from build123d import *

# Parameters (mm, degrees)
SKETCH1_W           = 260
SKETCH1_H           = 116
BOSS_EXTRUDE1_DEPTH = 75
SKETCH2_R           = 26.5
SKETCH2_W           = 191
SKETCH2_H           = 29
SKETCH2_H_2         = 77
SKETCH2_W_2         = 60
SKETCH2_H_3         = 25.123653406
SKETCH2_H_4         = 25.23272894
CUT_EXTRUDE1_DEPTH  = 69
FILLET1_R           = 5
FILLET2_R           = 5
SKETCH4_W           = 11.43
SKETCH4_H           = 4
CUT_EXTRUDE3_DEPTH  = 26.67
FILLET3_R           = 3
SKETCH5_W           = 55
SKETCH5_H           = 3
CUT_EXTRUDE4_DEPTH  = 1.5
SKETCH6_W           = 55
SKETCH6_H           = 3
CUT_EXTRUDE5_DEPTH  = 1.5
FILLET4_R           = 3
SKETCH7_W           = 162.299
SKETCH7_H           = 39.878
CUT_EXTRUDE6_DEPTH  = 10
SKETCH9_W           = 20
SKETCH9_H           = 3
CUT_EXTRUDE7_DEPTH  = 14.7
SKETCH10_W          = 3
SKETCH10_H          = 15.6
CUT_EXTRUDE8_DEPTH  = 22.8
SKETCH11_W          = 3
SKETCH11_H          = 22.8
BOSS_EXTRUDE2_DEPTH = 6.5
SKETCH12_W          = 15.39
SKETCH12_H          = 22.8
BOSS_EXTRUDE3_DEPTH = 3
SKETCH13_R          = 12.5
CUT_EXTRUDE9_DEPTH  = 3


with BuildPart() as part:
    # Sketch1 → Boss-Extrude1 (new body)
    with BuildSketch(Plane(origin=(0, 0, 0), x_dir=(1, 0, 0), z_dir=(0, 1, 0))):
        with Locations((130, 58)):
            Rectangle(SKETCH1_W, SKETCH1_H)
    extrude(amount=BOSS_EXTRUDE1_DEPTH)

    # Sketch2 → Cut-Extrude1 (cut)
    with BuildSketch(Plane(origin=(0, 75, 0), x_dir=(1, 0, 0), z_dir=(0, 1, 0))):
        with Locations((35, 58)):
            Circle(SKETCH2_R)
        with Locations((161.5, 98.5)):
            Rectangle(SKETCH2_W, SKETCH2_H)
        with Locations((161.5, 41.5)):
            Rectangle(SKETCH2_W, SKETCH2_H_2)
        with Locations((33, 100.438173297)):
            Rectangle(SKETCH2_W_2, SKETCH2_H_3)
        with Locations((33, 15.61636447)):
            Rectangle(SKETCH2_W_2, SKETCH2_H_4)
    extrude(amount=-CUT_EXTRUDE1_DEPTH, mode=Mode.SUBTRACT)

    # Fillet1
    fillet1_edges = [part.edges().sort_by_distance(p)[0] for p in [
        (0, 37.5, -116),
        (260, 37.5, -116),
        (260, 37.5, 0),
        (0, 37.5, 0),
    ]]
    fillet(fillet1_edges, radius=FILLET1_R)

    # Fillet2
    fillet2_edges = [part.edges().sort_by_distance(p)[0] for p in [
        (130, 0, -116),
        (0, 0, -58),
        (260, 0, -58),
        (130, 0, 0),
        (1.464466094, 0, -114.535533906),
        (1.464466094, 0, -1.464466094),
        (258.535533906, 0, -1.464466094),
        (258.535533906, 0, -114.535533906),
    ]]
    fillet(fillet2_edges, radius=FILLET2_R)

    # Sketch4 → Cut-Extrude3 (cut)
    with BuildSketch(Plane(origin=(0, 75, 0), x_dir=(1, 0, 0), z_dir=(0, 1, 0))):
        with Locations((180.625, 82)):
            Rectangle(SKETCH4_W, SKETCH4_H)
    extrude(amount=-CUT_EXTRUDE3_DEPTH, mode=Mode.SUBTRACT)

    # Fillet3
    fillet3_edges = [part.edges().sort_by_distance(p)[0] for p in [
        (186.34, 48.33, -82),
        (174.91, 48.33, -82),
        (186.34, 75, -82),
        (174.91, 75, -82),
    ]]
    fillet(fillet3_edges, radius=FILLET3_R)

    # Sketch5 → Cut-Extrude4 (cut)
    with BuildSketch(Plane.XY):
        with Locations((49.5, 69.5)):
            Rectangle(SKETCH5_W, SKETCH5_H)
        with Locations((210.5, 69.5)):
            Rectangle(SKETCH5_W, SKETCH5_H)
    extrude(amount=-CUT_EXTRUDE4_DEPTH, mode=Mode.SUBTRACT)

    # Sketch6 → Cut-Extrude5 (cut)
    with BuildSketch(Plane(origin=(0, 0, -116), x_dir=(-1, 0, 0), z_dir=(0, 0, -1))):
        with Locations((-210.5, 69.5)):
            Rectangle(SKETCH6_W, SKETCH6_H)
        with Locations((-49.5, 69.5)):
            Rectangle(SKETCH6_W, SKETCH6_H)
    extrude(amount=-CUT_EXTRUDE5_DEPTH, mode=Mode.SUBTRACT)

    # Fillet4
    fillet4_edges = [part.edges().sort_by_distance(p)[0] for p in [
        (3, 40.5, -87.876346594),
        (3, 40.5, -113),
        (63, 40.5, -113),
        (63, 40.5, -87.876346594),
        (3, 40.5, -3),
        (3, 40.5, -28.23272894),
        (63, 40.5, -28.23272894),
        (63, 40.5, -3),
    ]]
    fillet(fillet4_edges, radius=FILLET4_R)

    # Sketch7 → Cut-Extrude6 (cut)
    with BuildSketch(Plane(origin=(0, 0, -116), x_dir=(-1, 0, 0), z_dir=(0, 0, -1))):
        with Locations((-161.4995, 28.391)):
            Rectangle(SKETCH7_W, SKETCH7_H)
    extrude(amount=-CUT_EXTRUDE6_DEPTH, mode=Mode.SUBTRACT)

    # Sketch9 → Cut-Extrude7 (cut)
    with BuildSketch(Plane(origin=(0, 75, 0), x_dir=(1, 0, 0), z_dir=(0, 1, 0))):
        with Locations((158.35, 1.5)):
            Rectangle(SKETCH9_W, SKETCH9_H)
    extrude(amount=-CUT_EXTRUDE7_DEPTH, mode=Mode.SUBTRACT)

    # Sketch10 → Cut-Extrude8 (cut)
    with BuildSketch(Plane(origin=(0, 75, 0), x_dir=(1, 0, 0), z_dir=(0, 1, 0))):
        with Locations((258.5, 56.81)):
            Rectangle(SKETCH10_W, SKETCH10_H)
    extrude(amount=-CUT_EXTRUDE8_DEPTH, mode=Mode.SUBTRACT)

    # Sketch11 → Boss-Extrude2 (add)
    with BuildSketch(Plane.ZY.offset(-257)):
        with Locations((-47.51, 63.6)):
            Rectangle(SKETCH11_W, SKETCH11_H)
        with Locations((-66.11, 63.6)):
            Rectangle(SKETCH11_W, SKETCH11_H)
    extrude(amount=BOSS_EXTRUDE2_DEPTH)

    # Sketch12 → Boss-Extrude3 (add)
    with BuildSketch(Plane.ZY.offset(-250.5)):
        with Locations((-72.305, 63.6)):
            Rectangle(SKETCH12_W, SKETCH12_H)
        with Locations((-41.315, 63.6)):
            Rectangle(SKETCH12_W, SKETCH12_H)
    extrude(amount=BOSS_EXTRUDE3_DEPTH)

    # Sketch13 → Cut-Extrude9 (cut)
    with BuildSketch(Plane(origin=(0, 6, 0), x_dir=(1, 0, 0), z_dir=(0, 1, 0))):
        with Locations((35, 58)):
            Circle(SKETCH13_R)
    extrude(amount=-CUT_EXTRUDE9_DEPTH, mode=Mode.SUBTRACT)


solid = part.part
Source: CAD feature listing. Evaluate the final solid. Frame: model axes, mm. A direction names the side the tool comes from. Round coordinates to 2 decimals unless told otherwise and drop trailing zeros. Loops run counter-clockwise (first coordinate to the right, second up) from the corner with the lowest first, then second, coordinate; pieces in that order, holes last. Notation, with made-up numbers: (-37, 69.5) - (-13, 69.5) arc R14 ccw to (-13, 85.5) - close; hole circle Ø4 at (-24, 29.5). An arc over 180 degrees is marked (long way). Write item = value, one per line. Start each with the question number.
Item 1: Material intervals for line 1 (X direction, y = 36, z = -58); line 2 (Z direction, x = 73.5, y = 71.5); line 3 (Z direction, x = 35.5, y = 44.5), sorted ascending.
Item 2: Section query A-A on x = 129. Output: boundary loops of the cut face in (y, z).
Item 3: Section query D-D on y = 39.5. Count the separate pieces of the cut face and the enclosed holes in it, plus the area to 3 significant figures.
Item 4: Section query B-B on z = -58. Output: boundary loops of the cut face in (x, y).
Item 5: First-contact query: pin 1 Ø0.9 at (y, z) = (37.5, -114) entering from +X; pin 2 Ø6 at (x, y) = (217.5, 60) entering from +Z; pin 3 Ø2.5 at (y, z) = (65.5, -1.5) entering from -X; pin 4 Ø6 at (x, z) = (90.5, -24.5) entering from +Y. Flat tips, straight axial feed; report the tip coordinate or a pass-through.
Item 6: Mould query, pull axis Z, two halves, no side actions, for faces 4 (the face through (247.5, 64, -41)), 5 (the face through (258, 40, -115)), 6 (the face through (3, 41, -100)), 7 (the face through (260, 40, -57)). Classes: released by +Z, released by -Z, zero draft, split by the parting line, or undercut.
Item 7: Reachability of faces 1 (the face through (2, 1, -59)), 2 (the face through (250.5, 64, -40)), 3 (the face through (250, 52.2, -43)) from +Z, -Z, +X, -X, +Y, -Y: full face, straight path, thin tool, end or side. Return the list, or none.
Results list:
q1.line_1 = 0 to 8.5, 61.5 to 66, 257 to 260
q1.line_2 = -116 to -113, -84 to -80, -3 to 0
q1.line_3 = -116 to -113, -87.88 to -84.5, -31.5 to -28.23, -3 to 0
q2.outline = (0, -111) arc R5 ccw to (5, -116) - (8.45, -116) - (8.45, -113) - (6, -113) - (6, -84) - (75, -84) - (75, -80) - (6, -80) - (6, -3) - (75, -3) - (75, 0) - (5, 0) arc R5 ccw to (0, -5) - close; (48.33, -116) - (75, -116) - (75, -113) - (48.33, -113) - close
q3.separate_pieces = 1
q3.enclosed_holes = 4
q3.area = 4,190 mm²
q4.outline = (0, 5) arc R5 ccw to (5, 0) - (255, 0) arc R5 ccw to (260, 5) - (260, 52.2) - (257, 52.2) - (257, 6) - (66, 6) - (66, 75) - (61.5, 75) - (61.5, 6) - (47.5, 6) - (47.5, 3) - (22.5, 3) - (22.5, 6) - (8.5, 6) - (8.5, 75) - (0, 75) - close
q5.pin_1 = 259.3
q5.pin_2 = 0
q5.pin_3 = 0.53
q5.pin_4 = 6
q6.face_4 = undercut
q6.face_5 = released by -Z
q6.face_6 = undercut
q6.face_7 = zero draft
q7.face_1 = +Z, -Z, -X, -Y
q7.face_2 = +Y
q7.face_3 = none
